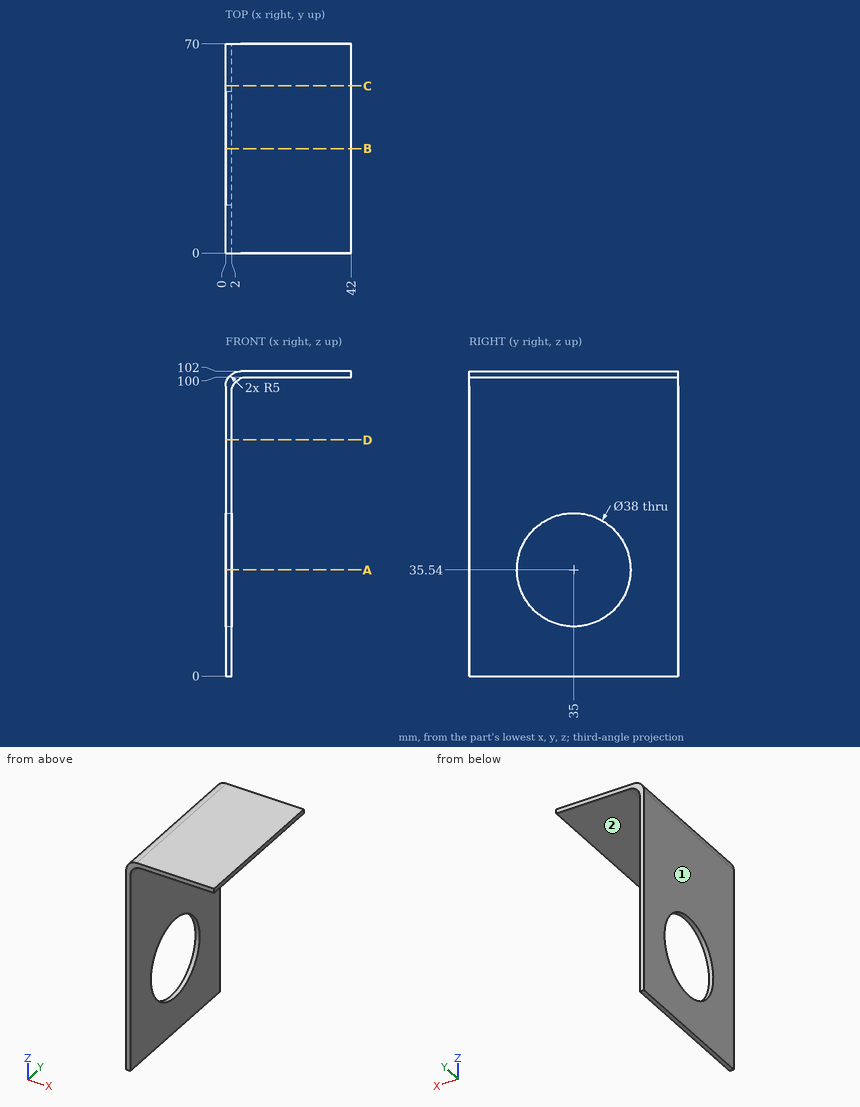
For this review, use the dimensioned drawing (mm, ordinates from the lowest corner) and the shaded views. A direction names the side the tool comes from. Round coordinates to 2 decimals unless told otherwise and drop trailing zeros. Order: outer loops, then holes, each group sorted by start corner. A loop starts at its lowest first (then second) coordinate and runs counter-clockwise, first axis right, second up. Notation, with made-up numbers: M -29.75,11 L -0.75,11 A21 ccw -0.75,50 Z; hole C -25,15.5 d9. An arc over 180 degrees is marked long. Use a Markdown table: item, result.
1) Insertion check: pin 1 (8 mm diameter, centred on x = 13, y = 50.5, fed in from -Z); pin 2 (5 mm diameter, centred on y = 62.5, z = 45.5, fed in from +X). Each pin has a flat end and moves straight along its axis. Give the tip position at first contact, or say it passes through.
Report:
| item | result |
|---|---|
| pin 1 | z = 100 |
| pin 2 | x = 2 |
2) Consider section C-C (y = 56). Write out the cut boundary in (x, z).
Report:
| item | result |
|---|---|
| outline | M 0,0 L 2,0 L 2,95 A5 cw 7,100 L 42,100 L 42,102 L 5,102 A5 ccw 0,97 Z |
3) Consider section A-A (z = 35.54). Write out the cut boundary in (x, y), then the cut area to 3 significant figures.
Report:
| item | result |
|---|---|
| outline | M 0,0 L 2,0 L 2,16 L 0,16 Z; M 0,54 L 2,54 L 2,70 L 0,70 Z |
| area | 64.0 mm^2 |
4) Tool access review of the marked faces 1 and 2: name each direction out of +Z, -Z, +X, -X, +Y, -Y from which nothing blocks a thin tool from reaching the whole face with its end or side.
Report:
| item | result |
|---|---|
| face 1 | +Z, -Z, -X, +Y, -Y |
| face 2 | -Z, +X, +Y, -Y |
5) Consider section D-D (z = 79). Write out the cut boundary in (x, y), then the cut area to 3 significant figures.
Report:
| item | result |
|---|---|
| outline | M 0,0 L 2,0 L 2,70 L 0,70 Z |
| area | 140 mm^2 |
6) Consider section B-B (y = 35). Write out the cut boundary in (x, z), then the cut area to 3 significant figures.
Report:
| item | result |
|---|---|
| outline | M 0,0 L 2,0 L 2,16.54 L 0,16.54 Z; M 0,54.54 L 2,54.54 L 2,95 A5 cw 7,100 L 42,100 L 42,102 L 5,102 A5 ccw 0,97 Z |
| area | 208 mm^2 |
7) Wall thickness on line 1 along Y through (x, z) = (0.7, 35.54); line 2 along Z through (x, y) = (28, 58); line 3 along X through (y, z) = (52, 71.5): over which ranges is each line inside the solid? List them lowest first. Write a range as [from, to].
Report:
| item | result |
|---|---|
| line 1 | [0, 16], [54, 70] |
| line 2 | [100, 102] |
| line 3 | [0, 2] |
